Geometry check sheet. Reference: the model listing, model coordinates, mm. A direction names the side the tool comes from. Coordinates: 2 decimals unless noted, no trailing zeros. Write each loop counter-clockwise with the first axis right and the second up, starting at its lowest first coordinate (ties: lowest second). Pieces come first, ordered by that corner, then holes. Notation, with made-up numbers: (-6, 20) -> (25, 20) arc R15 ccw to (25, 43) -> close; hole circle Ø11 at (54, 81). An arc over 180 degrees is marked (long way). Answer as CSV lines item,"result".
```python
from build123d import *

# Parameters (mm, degrees)
SKETCH1_W           = 50
SKETCH1_H           = 20
BOSS_EXTRUDE1_DEPTH = 5
SKETCH2_R           = 4
CUT_EXTRUDE1_DEPTH  = 5
SKETCH3_W           = 10
SKETCH3_H           = 20
BOSS_EXTRUDE2_DEPTH = 8
FILLET1_R           = 2
SKETCH5_W           = 20
SKETCH5_H           = 18
BOSS_EXTRUDE3_DEPTH = 5
SKETCH6_R           = 4
CUT_EXTRUDE2_DEPTH  = 5
FILLET2_R           = 2
BOSS_EXTRUDE4_DEPTH = 2


with BuildPart() as part:
    # Sketch1 → Boss-Extrude1 (new body)
    with BuildSketch(Plane(origin=(0, 0, 0), x_dir=(1, 0, 0), z_dir=(0, 1, 0))):
        Rectangle(SKETCH1_W, SKETCH1_H)
    boss_extrude1 = extrude(amount=BOSS_EXTRUDE1_DEPTH)

    # Sketch2 → Cut-Extrude1 (cut)
    with BuildSketch(Plane(origin=(0, 5, 0), x_dir=(1, 0, 0), z_dir=(0, 1, 0))):
        with Locations(Location((-15, 0, 0), (0, 0, 270))):
            Circle(SKETCH2_R)
        with Locations(Location((15, 0, 0), (0, 0, 270))):
            Circle(SKETCH2_R)
    cut_extrude1 = extrude(amount=-CUT_EXTRUDE1_DEPTH, mode=Mode.SUBTRACT)

    # Sketch3 → Boss-Extrude2 (add)
    with BuildSketch(Plane(origin=(0, 5, 0), x_dir=(1, 0, 0), z_dir=(0, 1, 0))):
        Rectangle(SKETCH3_W, SKETCH3_H)
    extrude(amount=BOSS_EXTRUDE2_DEPTH)

    # Mirror1: Boss-Extrude1, Cut-Extrude1 across plane
    add(boss_extrude1.mirror(Plane.ZX.offset(9)))
    add(cut_extrude1.mirror(Plane.ZX.offset(9)), mode=Mode.SUBTRACT)

    # Fillet1
    fillet1_edges = [part.edges().sort_by_distance(p)[0] for p in [
        (-25, 15.5, 10),
        (-25, 15.5, -10),
        (25, 15.5, -10),
        (25, 15.5, 10),
        (-25, 2.5, -10),
        (25, 2.5, -10),
        (25, 2.5, 10),
        (-25, 2.5, 10),
    ]]
    fillet(fillet1_edges, radius=FILLET1_R)

    # Sketch5 → Boss-Extrude3 (add)
    with BuildSketch(Plane.XY.offset(-10)):
        with Locations((0, 9)):
            Rectangle(SKETCH5_W, SKETCH5_H)
    extrude(amount=-BOSS_EXTRUDE3_DEPTH)

    # Sketch6 → Cut-Extrude2 (cut)
    with BuildSketch(Plane(origin=(0, 0, -15), x_dir=(-1, 0, 0), z_dir=(0, 0, -1))):
        with Locations((0, 9)):
            Circle(SKETCH6_R)
    extrude(amount=-CUT_EXTRUDE2_DEPTH, mode=Mode.SUBTRACT)

    # Fillet2
    fillet2_edges = [part.edges().sort_by_distance(p)[0] for p in [
        (10, 15.5, -10),
        (-10, 15.5, -10),
        (-10, 2.5, -10),
        (10, 2.5, -10),
        (5, 9, -10),
        (-5, 9, -10),
    ]]
    fillet(fillet2_edges, radius=FILLET2_R)

    # Sketch2_5 → Boss-Extrude4 (add)
    with BuildSketch(Plane(origin=(0, 5, 0), x_dir=(1, 0, 0), z_dir=(0, 1, 0))):
        Polygon((-5, -10), (-5, 0), (-8.48, -10), align=None)
        Polygon((5, 0), (5, -10), (8.48, -10), align=None)
    extrude(amount=BOSS_EXTRUDE4_DEPTH)


solid = part.part
```
Item 1: Cross-section at A-A, the plane y = 3. Record the cut outline in (x, z).
Responses:
outline,"(-25, -8) arc R2 ccw to (-23, -10) -> (-12, -10) arc R2 cw to (-10, -12) -> (-10, -15) -> (10, -15) -> (10, -12) arc R2 cw to (12, -10) -> (23, -10) arc R2 ccw to (25, -8) -> (25, 8) arc R2 ccw to (23, 10) -> (-23, 10) arc R2 ccw to (-25, 8) -> close; hole circle Ø8 at (-15, 0); hole circle Ø8 at (15, 0)"
Item 2: Cross-section at D-D, the plane z = -2.5. Record the cut outline in (x, y).
Responses:
outline,"(-25, 0) -> (-18.12, 0) -> (-18.12, 5) -> (-25, 5) -> close; (-25, 13) -> (-18.12, 13) -> (-18.12, 18) -> (-25, 18) -> close; (-11.88, 0) -> (11.88, 0) -> (11.88, 5) -> (5, 5) -> (5, 13) -> (11.88, 13) -> (11.88, 18) -> (-11.88, 18) -> (-11.88, 13) -> (-5, 13) -> (-5, 5) -> (-11.88, 5) -> close; (18.12, 0) -> (25, 0) -> (25, 5) -> (18.12, 5) -> close; (18.12, 13) -> (25, 13) -> (25, 18) -> (18.12, 18) -> close"
Item 3: Cross-section at B-B, the plane x = -20. Record the cut outline in (y, z), plus the area to 3 significant figures.
Responses:
outline,"(0, -10) -> (5, -10) -> (5, 10) -> (0, 10) -> close; (13, -10) -> (18, -10) -> (18, 10) -> (13, 10) -> close"
area,"200 mm2"
Item 4: Thickness scan on probe 1 along Y at (x, z) = (0, -11.6); probe 2 along X at (y, z) = (15.5, 0); probe 3 along X at (y, z) = (14, -12.75). Record the ranges inside material, lowest first.
Responses:
probe 1,"y = 0 to 5, 13 to 18"
probe 2,"x = -25 to -19, -11 to 11, 19 to 25"
probe 3,"x = -10 to 10"
Item 5: Depth check by flat-ended pin: pin 1 Ø1.5 at (x, y) = (20, 2) entering from -Z; pin 2 Ø0.9 at (x, y) = (-8, 7.5) entering from +Z; pin 3 Ø2.5 at (y, z) = (8, -1) entering from -X. Enter the tip coordinate at first touch or a pass-through.
Responses:
pin 1,"stops at z = -10"
pin 2,"stops at z = -10"
pin 3,"stops at x = -5"
Item 6: Release check for a two-part mould opening along Z. For faces 1 (the cylindrical face through (-11.034, 2.535, -0.521)), 2 (the cylindrical face through (18.966, 15.465, -0.521)), 3 (the flat face through (25, 2, 0)), 4 (the flat face through (17, 3, -10)) record: +Z half, -Z half, draft (parallel to the pull), parting line (faces both ways), or undercut.
Responses:
face 1,"undercut"
face 2,"undercut"
face 3,"draft"
face 4,"-Z half"
Item 7: Cross-section at C-C, the plane x = 15. Record the cut outline in (y, z).
Responses:
outline,"(0, -10) -> (5, -10) -> (5, -4) -> (0, -4) -> close; (0, 4) -> (5, 4) -> (5, 10) -> (0, 10) -> close; (13, -10) -> (18, -10) -> (18, -4) -> (13, -4) -> close; (13, 4) -> (18, 4) -> (18, 10) -> (13, 10) -> close"
Item 8: Set-up check for faces 5 (the flat face through (-6.716, 5.986, 4.93)), 6 (the flat face through (17, 5, -4)), 7 (the cylindrical face through (0.867, 5.095, -12.535)), 8 (the flat face through (-17, 13, -4)): record each of +Z, -Z, +X, -X, +Y, -Y from which the full face is reachable in a straight line by a thin tool's end or side.
Responses:
face 5,"-X"
face 6,"+X"
face 7,"-Z"
face 8,"+Z, -X"
